Model file for the job. Use its own axes, mm. Coordinates: 2 decimals unless noted, no trailing zeros. Write each loop counter-clockwise with the first axis right and the second up, starting at its lowest first coordinate (ties: lowest second). Pieces come first, ordered by that corner, then holes. Notation, with made-up numbers: M 45.5,-29.5 L 101.5,-29.5 A28 cw 101.5,5.5 Z; hole C 85,32 d9. An arc over 180 degrees is marked long. One line per question, with ' | ' between items. Start each with the question number.
(1) Wall check: probe 1 along X at (y, z) = (-10.75, -0.5); probe 2 along Z at (x, y) = (1.5, -13.5); probe 3 along X at (y, z) = (-18.5, -3). Give the ranges that are in metal, low to high.
(2) Cut at B-B (x = -36). Write the cut outline in (y, z), plus the area to 3 significant figures.
(3) Cut at D-D (y = -7). Count the separate pieces of the cut face and the enclosed holes in it, plus the area to 3 significant figures.
(4) Flat gauge pins, fed straight in: pin 1 Ø2 at (x, y) = (26.5, -15) entering from -Z; pin 2 Ø6 at (y, z) = (-5.5, 34.5) entering from +X; pin 3 Ø10.5 at (x, z) = (0, -35) entering from -Y; pin 4 Ø1.5 at (x, y) = (-24.5, -5) entering from -Z. Where does each tip first touch, or does it go through?
(5) Cut at A-A (z = 0). Write the cut outline in (x, y).
(6) Cut at C-C (z = -35). Write the cut outline in (x, y).
from build123d import *

# Parameters (mm, degrees)
F0_R     = 50
F0_R_2   = 4
F1_DEPTH = 25


with BuildPart() as f1:
    # F0 (on Front) → F1 (new body)
    with BuildSketch(Plane.XZ):
        Circle(F0_R)
        with Locations((-24.748737, -24.748737)):
            Circle(F0_R_2, mode=Mode.SUBTRACT)
        with Locations((0, -35)):
            Circle(F0_R_2, mode=Mode.SUBTRACT)
        with Locations((24.748737, -24.748737)):
            Circle(F0_R_2, mode=Mode.SUBTRACT)
        with Locations((-35, 0)):
            Circle(F0_R_2, mode=Mode.SUBTRACT)
        with Locations((-24.748737, 24.748737)):
            Circle(F0_R_2, mode=Mode.SUBTRACT)
        with Locations((24.748737, 24.748737)):
            Circle(F0_R_2, mode=Mode.SUBTRACT)
        with Locations((35, 0)):
            Circle(F0_R_2, mode=Mode.SUBTRACT)
        with Locations((0, 35)):
            Circle(F0_R_2, mode=Mode.SUBTRACT)
    extrude(amount=F1_DEPTH)


solid = f1.part
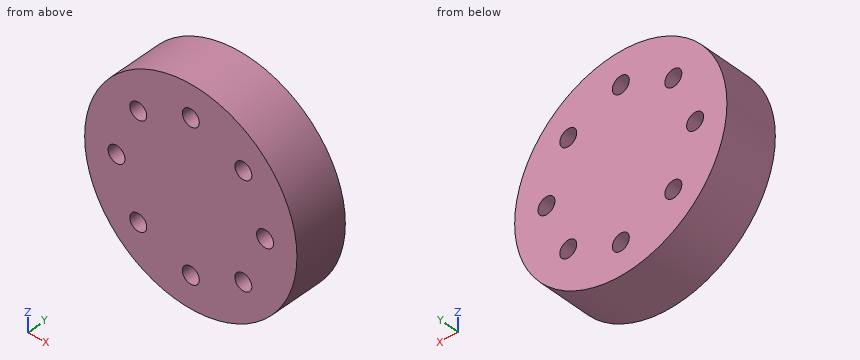
Filled in:
1) probe 1: -50 to -38.97, -31.03 to 31.03, 38.97 to 50 | probe 2: -49.98 to -38.71, -31.29 to 31.29, 38.71 to 49.98 | probe 3: -49.91 to -37.65, -32.35 to 32.35, 37.65 to 49.91
2) outline: M -25,-34.7 L 0,-34.7 L 0,-3.87 L -25,-3.87 Z; M -25,3.87 L 0,3.87 L 0,34.7 L -25,34.7 Z | area: 1,540 mm²
3) separate pieces: 1 | enclosed holes: 8 | area: 7,450 mm²
4) pin 1: z = -43.01 | pin 2: x = 38.83 | pin 3: y = -25 | pin 4: z = -44
5) outline: M -50,-25 L -39,-25 L -39,0 L -50,0 Z; M -31,-25 L 31,-25 L 31,0 L -31,0 Z; M 39,-25 L 50,-25 L 50,0 L 39,0 Z
6) outline: M -35.71,-25 L -4,-25 L -4,0 L -35.71,0 Z; M 4,-25 L 35.71,-25 L 35.71,0 L 4,0 Z
